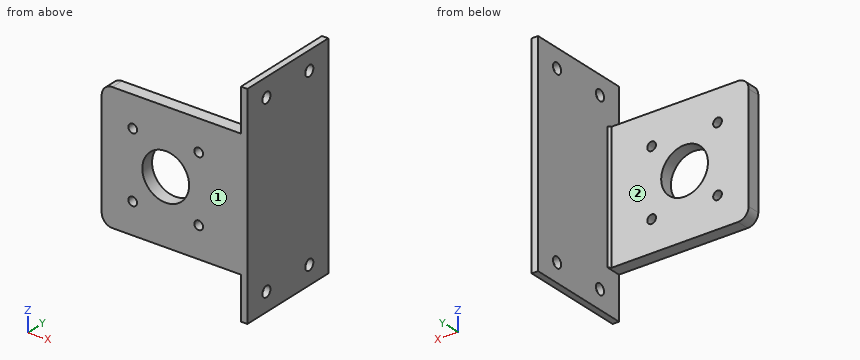
from build123d import *

# Parameters (mm, degrees)
EXTRUDE_1_DEPTH     = 60
SKETCH_4_R          = 11
SKETCH_4_R_2        = 2.05
CUT_EXTRUDE_3_DEPTH = 7
FILLET_2_R          = 5
SKETCH_5_W          = 100
SKETCH_5_H          = 50
SKETCH_5_R          = 2.5
EXTRUDE_2_DEPTH     = 3


with BuildPart() as part:
    # 草图1 → 凸台-拉伸1 (new body)
    with BuildSketch(Plane.XY):
        Polygon((0, 0), (68.5, 0), (68.5, 50), (65.5, 50), (65.5, 7), (64.5, 6), (0, 6), align=None)
    extrude(amount=EXTRUDE_1_DEPTH)

    # 草图4 → 切除-拉伸3 (cut, through all)
    with BuildSketch(Plane(origin=(0, 6, 0), x_dir=(1, 0, 0), z_dir=(0, 1, 0))):
        with Locations((30.1, -30)):
            Circle(SKETCH_4_R)
        with Locations((14.6, -14.5)):
            Circle(SKETCH_4_R_2)
        with Locations((45.6, -14.5)):
            Circle(SKETCH_4_R_2)
        with Locations((45.6, -45.5)):
            Circle(SKETCH_4_R_2)
        with Locations((14.6, -45.5)):
            Circle(SKETCH_4_R_2)
    extrude(amount=-CUT_EXTRUDE_3_DEPTH, mode=Mode.SUBTRACT)

    # 圆角2
    fillet_2_edges = [part.edges().sort_by_distance(p)[0] for p in [
        (0, 3, 0),
        (0, 3, 60),
    ]]
    fillet(fillet_2_edges, radius=FILLET_2_R)

    # 草图5 → 凸台-拉伸2 (add)
    with BuildSketch(Plane.ZY.offset(-65.5)):
        with Locations((30, 25)):
            Rectangle(SKETCH_5_W, SKETCH_5_H)
        with Locations((71.25, 11.75)):
            Circle(SKETCH_5_R, mode=Mode.SUBTRACT)
        with Locations((-11.25, 11.75)):
            Circle(SKETCH_5_R, mode=Mode.SUBTRACT)
        with Locations((-11.25, 38.25)):
            Circle(SKETCH_5_R, mode=Mode.SUBTRACT)
        with Locations((71.25, 38.25)):
            Circle(SKETCH_5_R, mode=Mode.SUBTRACT)
    extrude(amount=-EXTRUDE_2_DEPTH)


solid = part.part
Could you check a few things on this model? Use its own coordinates, in mm. Face numbers are marked on the shaded views. A direction names the side the tool comes from. Give positions to 0.01 mm unless a question says otherwise; leave off trailing zeros. Loops run counter-clockwise (first coordinate to the right, second up) from the corner with the lowest first, then second, coordinate; pieces in that order, holes last. Notation, with made-up numbers: (58, 1.25) -> (92, 1.25) arc R10 cw to (92, 17.25) -> close; hole circle Ø1 at (-27, -39.75). An arc over 180 degrees is marked (long way). Return JSON: item names as keys, results as strings.
Item 1: I need wall thicknesses on L1, parallel to Y at x = 66.6, z = -11.25; L2, parallel to X at y = 3.4, z = 45.5; L3, parallel to Z at x = 30, y = 3. Which ranges of each line are inside material? Lowest first, please. Write a range as from..to.
Geometry results:
{"L1": "y = 0..9.25, 14.25..35.75, 40.75..50", "L2": "x = 0..12.55, 16.65..43.55, 47.65..68.5", "L3": "z = 0..19, 41..60"}
Item 2: If we section it at D-D on x = 30.1: List the corners of the cut face in (y, z) for me, plus the area to 3 significant figures.
Geometry results:
{"outline": "(0, 0) -> (6, 0) -> (6, 19) -> (0, 19) -> close; (0, 41) -> (6, 41) -> (6, 60) -> (0, 60) -> close", "area": "228 mm²"}
Item 3: If we section it at C-C on y = 38.25: List the corners of the cut face in (x, z) for me, plus the area to 3 significant figures.
Geometry results:
{"outline": "(65.5, -20) -> (68.5, -20) -> (68.5, -13.75) -> (65.5, -13.75) -> close; (65.5, -8.75) -> (68.5, -8.75) -> (68.5, 68.75) -> (65.5, 68.75) -> close; (65.5, 73.75) -> (68.5, 73.75) -> (68.5, 80) -> (65.5, 80) -> close", "area": "270 mm²"}
Item 4: If we section it at A-A on x = 14.6: List the corners of the cut face in (y, z) for me.
Geometry results:
{"outline": "(0, 0) -> (6, 0) -> (6, 12.45) -> (0, 12.45) -> close; (0, 16.55) -> (6, 16.55) -> (6, 43.45) -> (0, 43.45) -> close; (0, 47.55) -> (6, 47.55) -> (6, 60) -> (0, 60) -> close"}
Item 5: If we section it at B-B on z = 30: List the corners of the cut face in (x, y) for me.
Geometry results:
{"outline": "(0, 0) -> (19.1, 0) -> (19.1, 6) -> (0, 6) -> close; (41.1, 0) -> (68.5, 0) -> (68.5, 50) -> (65.5, 50) -> (65.5, 7) -> (64.5, 6) -> (41.1, 6) -> close"}
Item 6: Which directions (+Z, -Z, +X, -X, +Y, -Y) give clear straight access to the entire face, cutting with the end or side of a thin tool? Please do the marked faces 1 and 2.
Geometry results:
{"face 1": "+Z, -Z, +X, -X, -Y", "face 2": "+Z, -Z, -X, +Y"}
Item 7: I'm going to push flat-ended pins straight in: pin 1 (4.5 mm diameter, centred on x = 14.6, z = 45.5, fed in from +Y); pin 2 (6 mm diameter, centred on y = 38.25, z = 71.25, fed in from -X); pin 3 (2 mm diameter, centred on x = 47.5, y = 3, fed in from -Z). Where does each tip first touch, or does it pass through?
Geometry results:
{"pin 1": "stops at y = 6", "pin 2": "stops at x = 65.5", "pin 3": "stops at z = 0"}
